The drawing under review shows one solid part. Ordinate dimensions are in mm from its lowest x, y, z. A direction names the side the tool comes from. Give positions to 0.01 mm unless a question says otherwise; leave off trailing zeros. Loops run counter-clockwise (first coordinate to the right, second up) from the corner with the lowest first, then second, coordinate; pieces in that order, holes last.
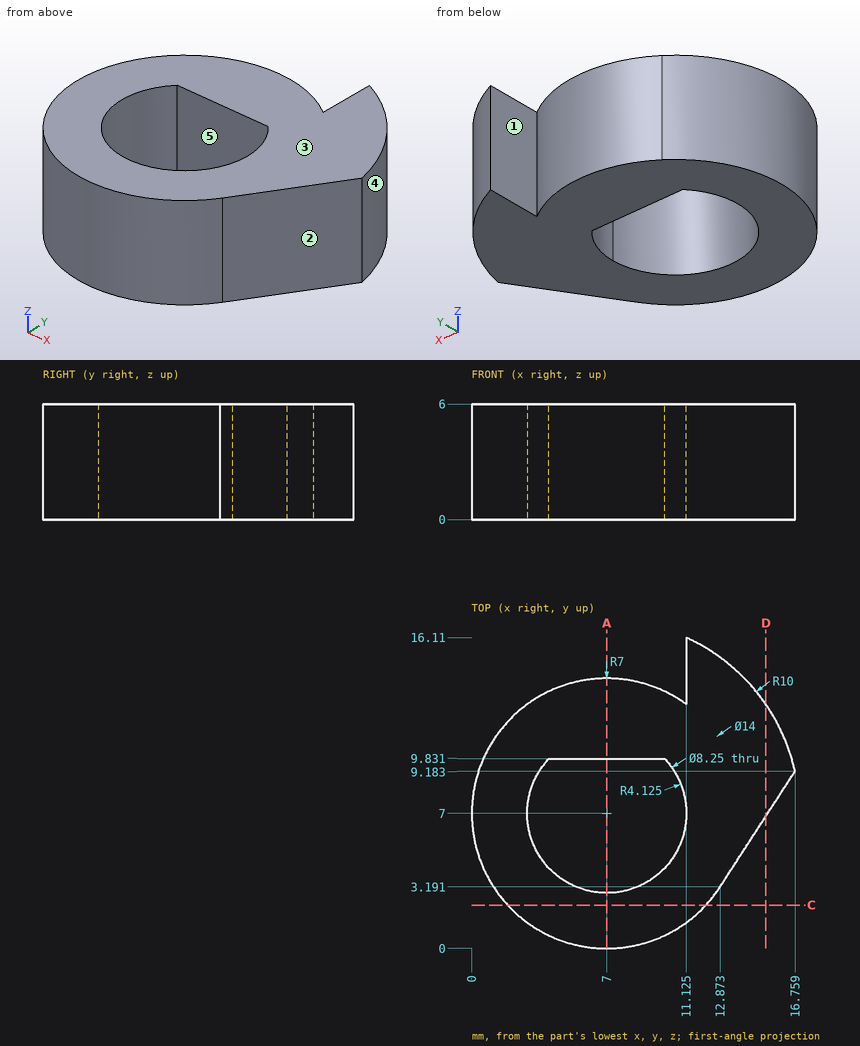
Item 1: Take a section at A-A on x = 7. Give the boundary of the cut face in (y, z) (1 decimal).
Answer:
outline: (0, 0) - (2.9, 0) - (2.9, 6) - (0, 6) - close; (9.8, 0) - (14, 0) - (14, 6) - (9.8, 6) - close
Item 2: Take a section at C-C on y = 2.25. Give the boundary of the cut face in (x, z).
Answer:
outline: (1.86, 0) - (12.14, 0) - (12.14, 6) - (1.86, 6) - close
Item 3: Clearance check with flat-ended pins moving along their axes: pin 1 Ø1 at (x, z) = (8.5, 4.5) entering from +Y; pin 2 Ø3 at (y, z) = (2.5, 1) entering from -X (1 decimal); pin 3 Ø2 at (x, z) = (9.5, 3.5) entering from +Y; pin 4 Ø2 at (x, y) = (9.5, 5.5) entering from +Z. State where each tip first meets the part, or that it passes through.
Answer:
pin 1: stops at y = 13.93
pin 2: stops at x = 0.7
pin 3: stops at y = 13.84
pin 4: passes through
Item 4: Tool access review of the marked faces 1 and 2: name each direction out of +Z, -Z, +X, -X, +Y, -Y from which nothing blocks a thin tool from reaching the whole face with its end or side.
Answer:
face 1: +Z, -Z, +Y
face 2: +Z, -Z, +X, -Y
Item 5: Take a section at D-D on x = 15.25. Give the boundary of the cut face in (y, z).
Answer:
outline: (6.86, 0) - (12.65, 0) - (12.65, 6) - (6.86, 6) - close
Item 6: The part is to be moulded in two halves that separate along X. For the marked faces 3, 4 and 5, say which applies: released by +X, released by -X, zero draft, split by the parting line, or undercut.
Answer:
face 3: zero draft
face 4: released by +X
face 5: undercut
Item 7: For L1, parallel to Y at x = 7, z = 2.8 (1 decimal); L2, parallel to X at y = 7, z = 4.75 (1 decimal); L3, parallel to Y at x = 9.75, z = 5.65 (1 decimal), list the stretches that pass through material, from the lowest coordinate up.
Answer:
L1: y = 0 to 2.9, 9.8 to 14
L2: x = 0 to 2.9, 11.1 to 15.3
L3: y = 0.6 to 3.9, 9.8 to 13.4
